Geometry check sheet. Reference: the model listing, model coordinates, mm. Face numbers are marked on the shaded views. A direction names the side the tool comes from. Give positions to 0.01 mm unless a question says otherwise; leave off trailing zeros. Write each loop counter-clockwise with the first axis right and the second up, starting at its lowest first coordinate (ties: lowest second). Pieces come first, ordered by that corner, then holes. Notation, with made-up numbers: (41.25, 73) - (85.25, 73) arc R24 ccw to (85.25, 99) - close; hole circle Ø11 at (-31.75, 83.5). An arc over 180 degrees is marked (long way). Use a Markdown table: item, result.
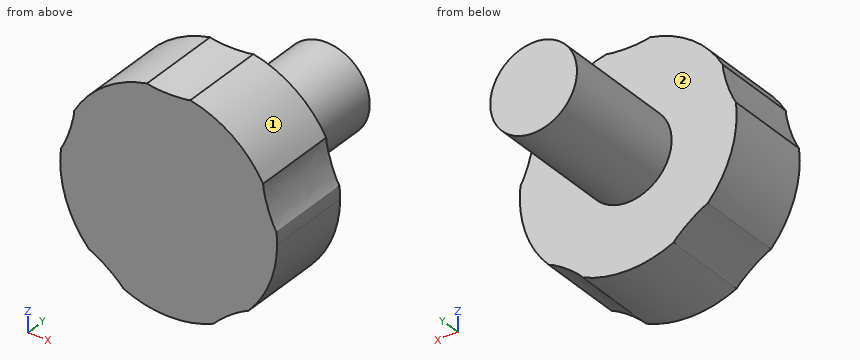
```python
from build123d import *

# Parameters (mm, degrees)
F0_R     = 5
F1_DEPTH = 25
F2_DEPTH = 10


with BuildPart() as f1:
    # F0 (on Front) → F1 (new body)
    with BuildSketch(Plane.XZ):
        Circle(F0_R)
    extrude(amount=-F1_DEPTH)

    # F0 (on Front) → F2 (join)
    with BuildSketch(Plane.XZ):
        with BuildLine():
            ThreePointArc((10.8845513989, 6.1462623475), (7.3547721112, 10.1072907939), (2.5, 12.2474487139))
            add(Edge.make_bspline(
                [(-2.5, 12.2474487139), (0, 11.5101020514), (2.5, 12.2474487139)],
                knots=[0.5295008084, 0.5295008084, 0.5295008084, 2.6120918452, 2.6120918452, 2.6120918452], degree=2, weights=[1, 0.5051025722, 1]))
            ThreePointArc((-2.5, 12.2474487139), (-7.3594746101, 10.1038672529), (-10.8902668496, 6.1361297203))
            add(Edge.make_bspline(
                [(-12.4183614967, 1.4262880979), (-10.9820454119, 3.5733899362), (-10.8902668496, 6.1361297203)],
                knots=[0.5483081022, 0.5483081022, 0.5483081022, 2.5982377345, 2.5982377345, 2.5982377345], degree=2, weights=[1, 0.5191289586, 1]))
            ThreePointArc((-12.4183614967, 1.4262880979), (-11.883327852, -3.8776950837), (-9.1869736579, -8.4764093228))
            add(Edge.make_bspline(
                [(-5.2222037532, -11.35687404), (-6.8105963999, -9.3736670378), (-9.1869736579, -8.4764093228)],
                knots=[0.5626274917, 0.5626274917, 0.5626274917, 2.5791740982, 2.5791740982, 2.5791740982], degree=2, weights=[1, 0.5333221495, 1]))
            ThreePointArc((-5.2222037532, -11.35687404), (-0.008685173, -12.4999969827), (5.2064168882, -11.3641199917))
            add(Edge.make_bspline(
                [(9.1879155932, -8.4753883128), (6.8082361023, -9.3588262471), (5.2064168882, -11.3641199917)],
                knots=[0.5527221385, 0.5527221385, 0.5527221385, 2.5812548422, 2.5812548422, 2.5812548422], degree=2, weights=[1, 0.5282430094, 1]))
            ThreePointArc((9.1879155932, -8.4753883128), (11.6425715569, -4.5497832413), (12.5, 0))
            ThreePointArc((12.5, 0), (12.4800818706, 0.7053768519), (12.4203909595, 1.4085057378))
            add(Edge.make_bspline(
                [(10.8845513989, 6.1462623475), (10.9593557736, 3.5694882441), (12.4203909595, 1.4085057378)],
                knots=[0.53219448, 0.53219448, 0.53219448, 2.6015416859, 2.6015416859, 2.6015416859], degree=2, weights=[1, 0.510806562, 1]))
        make_face()
        Circle(F0_R, mode=Mode.SUBTRACT)
    extrude(amount=-F2_DEPTH)


solid = f1.part
```
1) Section check B-B on z = 7.25. Record the boundary of the cut face in (x, y), then the cut area to 3 significant figures.
Working result:
| item | result |
|---|---|
| outline | (-10.18, 0) - (10.18, 0) - (10.18, 10) - (-10.18, 10) - close |
| area | 204 mm² |
2) Depth check by flat-ended pin: P1, Ø4, axis at x = -3.5, y = 15.5, coming from the +Z side; P2, Ø3, axis at y = 20, z = 4.5, coming from the +X side; P3, Ø1, axis at x = -1.5, y = 8, coming from the -Z side. Enter the tip coordinate at first touch or a pass-through.
Working result:
| item | result |
|---|---|
| P1 | stops at z = 4.77 |
| P2 | stops at x = 4 |
| P3 | stops at z = -12.46 |
3) Set-up check for the marked faces 1 and 2: record each of +Z, -Z, +X, -X, +Y, -Y from which the full face is reachable in a straight line by a thin tool's end or side.
Working result:
| item | result |
|---|---|
| face 1 | +Z, +X, +Y, -Y |
| face 2 | +Y |
4) Section check C-C on x = -10.5. Record the boundary of the cut face in (y, z), then the cut area to 3 significant figures.
Working result:
| item | result |
|---|---|
| outline | (0, -6.78) - (10, -6.78) - (10, 6.78) - (0, 6.78) - close |
| area | 136 mm² |
5) Material ranges on L1, parallel to Y at x = -0.75, z = 9.75; L2, parallel to X at y = 22.5, z = -3.5; L3, parallel to X at y = 3.75, z = -4.25, recorded low to high. Write a range as from..to.
Working result:
| item | result |
|---|---|
| L1 | y = 0..10 |
| L2 | x = -3.57..3.57 |
| L3 | x = -11.76..11.76 |
6) Section check A-A on y = 23.25. Record the boundary of the cut face in (x, z), then the cut area to 3 significant figures.
Working result:
| item | result |
|---|---|
| outline | circle Ø10 at (0, 0) |
| area | 78.5 mm² |
